Verification items for the finished model (mm, model axes). Face numbers are marked on the shaded views. A direction names the side the tool comes from. Coordinates: 2 decimals unless noted, no trailing zeros. Write each loop counter-clockwise with the first axis right and the second up, starting at its lowest first coordinate (ties: lowest second). Pieces come first, ordered by that corner, then holes. Notation, with made-up numbers: M 21,70.5 L 42,70.5 A32 cw 42,96.5 Z; hole C -27.75,86.25 d1. An arc over 180 degrees is marked long. Answer in a Markdown table with one row per item.
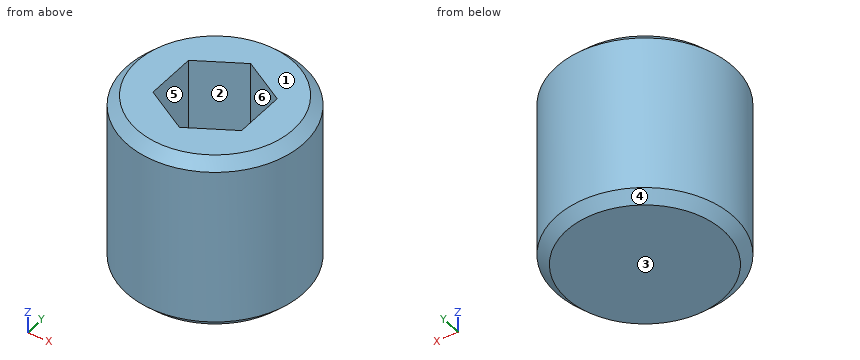
from build123d import *

# Parameters (mm, degrees)
SZKIC3_R                    = 3.009401077
DODANIE_WYCI_GNI_CIE1_DEPTH = 6


with BuildPart() as part:
    # Szkic1 → Obrót1 (revolve)
    with BuildSketch(Plane(origin=(0, 0, 0), x_dir=(0, 0, -1), z_dir=(1, 0, 0)), mode=Mode.PRIVATE) as obr_t1_sk:
        Polygon((-8, 0), (-8, 3.54), (-7.54, 4), (-0.46, 4), (0, 3.54), (0, 0), align=None)
    revolve(obr_t1_sk.sketch.rotate(Axis((0, 0, 0), (0, 0, 1)), 270), axis=Axis((0, 0, 0), (0, 0, 1)))

    # Szkic2 → Wycięcie-obrót1 (revolve, cut)
    with BuildSketch(Plane(origin=(0, 0, 0), x_dir=(0, 0, -1), z_dir=(1, 0, 0)), mode=Mode.PRIVATE) as wyci_cie_obr_t1_sk:
        Polygon((-8, 0), (-8, 2.809401077), (-4, 2.809401077), (-2.377991532, 0), align=None)
    revolve(wyci_cie_obr_t1_sk.sketch.rotate(Axis((0, 0, 2.377991532), (0, 0, 1)), 270), axis=Axis((0, 0, 2.377991532), (0, 0, 1)), mode=Mode.SUBTRACT)

    # Szkic3 → Dodanie-wyciągnięcie1 (add)
    with BuildSketch(Plane.XY.offset(8)):
        Circle(SZKIC3_R)
        Polygon((-2, 1.154700538), (-2, -1.154700538), (0, -2.309401077), (2, -1.154700538), (2, 1.154700538), (0, 2.309401077), align=None, mode=Mode.SUBTRACT)
    extrude(amount=-DODANIE_WYCI_GNI_CIE1_DEPTH)


solid = part.part
1) Sectioned sample at A-A (z = 4). Record the cut outline in (x, y).
Response values:
| item | result |
|---|---|
| outline | C 0,0 d8; hole M -2,-1.15 L 0,-2.31 L 2,-1.15 L 2,1.15 L 0,2.31 L -2,1.15 Z |
2) Sectioned sample at B-B (z = 2). Record the cut outline in (x, y).
Response values:
| item | result |
|---|---|
| outline | C 0,0 d8 |
3) Release check for a two-part mould opening along X. For the marked faces 3, 4, 5 and 6 record: +X half, -X half, draft (parallel to the pull), parting line (faces both ways), or undercut.
Response values:
| item | result |
|---|---|
| face 3 | draft |
| face 4 | parting line |
| face 5 | undercut |
| face 6 | undercut |
4) Thickness scan on L1, parallel to Y at x = -0.75, z = 7.5; L2, parallel to Y at x = 1, z = 5.75; L3, parallel to X at y = -1.75, z = 5.5. Record the ranges inside material, lowest first. Write a range as [from, to].
Response values:
| item | result |
|---|---|
| L1 | y = [-3.93, -1.88], [1.88, 3.93] |
| L2 | y = [-3.87, -1.73], [1.73, 3.87] |
| L3 | x = [-3.6, -0.97], [0.97, 3.6] |
5) Tool access check on the marked faces 1 and 2. Record the directions out of +Z, -Z, +X, -X, +Y, -Y that give a thin tool (end or side, any length) a straight path to the whole face; none if there is none.
Response values:
| item | result |
|---|---|
| face 1 | +Z, +X, -X, +Y, -Y |
| face 2 | +Z |
